Part model, mm, in its own coordinate system. Face numbers are marked on the shaded views. A direction names the side the tool comes from. Coordinates: 2 decimals unless noted, no trailing zeros. Order: outer loops, then holes, each group sorted by start corner. A loop starts at its lowest first (then second) coordinate and runs counter-clockwise, first axis right, second up. Notation, with made-up numbers: M 72.25,79.25 L 90.25,79.25 A19 ccw 90.25,111.25 Z; hole C 17,84.5 d8. An arc over 180 degrees is marked long. Write item = value, one per line. Start each with the question number.
from build123d import *

# Parameters (mm, degrees)
SKETCH007_W      = 1.5
SKETCH007_H      = 1
EXTRUDE008_DEPTH = 1
BOX004_W         = 8
BOX004_H         = 8
BOX004_DEPTH     = 1


with BuildPart() as wedgeextrude:
    # Sketch007 (on Face6 of Box004) → Extrude008 (new body)
    with BuildSketch(Plane(origin=(43.86, 17.4167, 1), x_dir=(1, 0, 0), z_dir=(0, 0, 1))):
        with BuildLine():
            Line((5.5, 8), (2.5, 8))
            Line((2.5, 10.414147), (2.5, 8))
            ThreePointArc((3.085853, 11), (2.671592, 10.828408), (2.5, 10.414147))
            Line((3.085853, 11), (4.914147, 11))
            ThreePointArc((5.5, 10.414147), (5.328408, 10.828408), (4.914147, 11))
            Line((5.5, 10.414147), (5.5, 8))
        make_face()
        with Locations((4, 9.5)):
            Rectangle(SKETCH007_W, SKETCH007_H, mode=Mode.SUBTRACT)
    extrude(amount=-EXTRUDE008_DEPTH)


with BuildPart() as wedgewedge:
    # Box004 → Box004 (new body)
    with BuildSketch(Plane(origin=(43.86, 17.4167, 0), x_dir=(1, 0, 0), z_dir=(0, 0, 1))):
        with Locations((4, 4)):
            Rectangle(BOX004_W, BOX004_H)
    extrude(amount=BOX004_DEPTH)

    # Fusion001: union wedgeExtrude
    add(wedgeextrude.part)


solid = wedgewedge.part
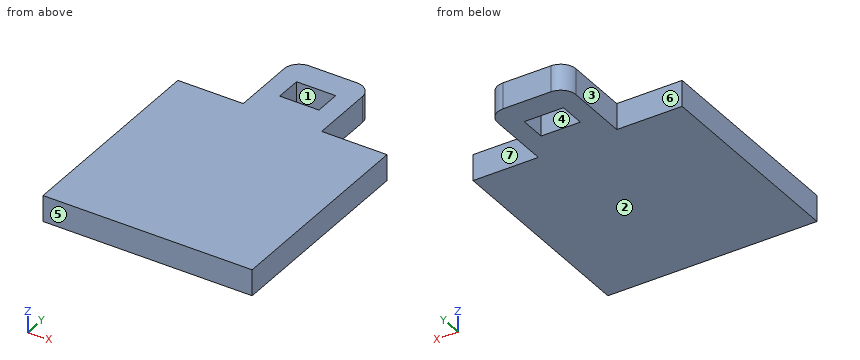
Item 1: Cut at D-D, the plane x = 46. Write the cut outline in (y, z).
Item 2: Cut at A-A, the plane x = 47.25. Write the cut outline in (y, z), and give its area (3 significant figures).
Item 3: 3-axis set-ups, long thin cutter, end or side, ignore diameter. For the marked faces 5, 6 and 7: which of +Z, -Z, +X, -X, +Y, -Y reach the whole face in a straight line?
Item 4: Cut at B-B, the plane z = 0.6. Write the cut outline in (x, y).
Item 5: Pull direction X, two halves, no side cores. Call the marked faces 1, 2, 3 and 4: pulls with the +X half, pulls with the -X half, needs draft (parallel to the pull), parting line crosses it, or undercut.
Item 6: Wall check: line 1 along Y through (x, z) = (47.5, 0.6); line 2 along X through (y, z) = (27.25, 0.45); line 3 along Y through (x, z) = (45, 0.45). Give the ranges that are in metal, low to high. Write a range as [from, to].
Item 7: Cut at C-C, the plane y = 27.25. Write the cut outline in (x, z), and give its area (3 significant figures).
Filled sheet:
q1.outline = M 17.42,0 L 25.42,0 L 25.42,1 L 17.42,1 Z
q2.outline = M 17.42,0 L 26.42,0 L 26.42,1 L 17.42,1 Z; M 27.42,0 L 28.42,0 L 28.42,1 L 27.42,1 Z
q2.area = 10.0 mm2
q3.face_5 = +Z, -Z, +X, -X, -Y
q3.face_6 = +Z, -Z, -X, +Y
q3.face_7 = +Z, -Z, +X, +Y
q4.outline = M 43.86,17.42 L 51.86,17.42 L 51.86,25.42 L 49.36,25.42 L 49.36,27.83 A0.59 ccw 48.77,28.42 L 46.95,28.42 A0.59 ccw 46.36,27.83 L 46.36,25.42 L 43.86,25.42 Z; hole M 47.11,26.42 L 48.61,26.42 L 48.61,27.42 L 47.11,27.42 Z
q5.face_1 = undercut
q5.face_2 = needs draft
q5.face_3 = pulls with the -X half
q5.face_4 = undercut
q6.line_1 = [17.42, 26.42], [27.42, 28.42]
q6.line_2 = [46.36, 47.11], [48.61, 49.36]
q6.line_3 = [17.42, 25.42]
q7.outline = M 46.36,0 L 47.11,0 L 47.11,1 L 46.36,1 Z; M 48.61,0 L 49.36,0 L 49.36,1 L 48.61,1 Z
q7.area = 1.50 mm2
